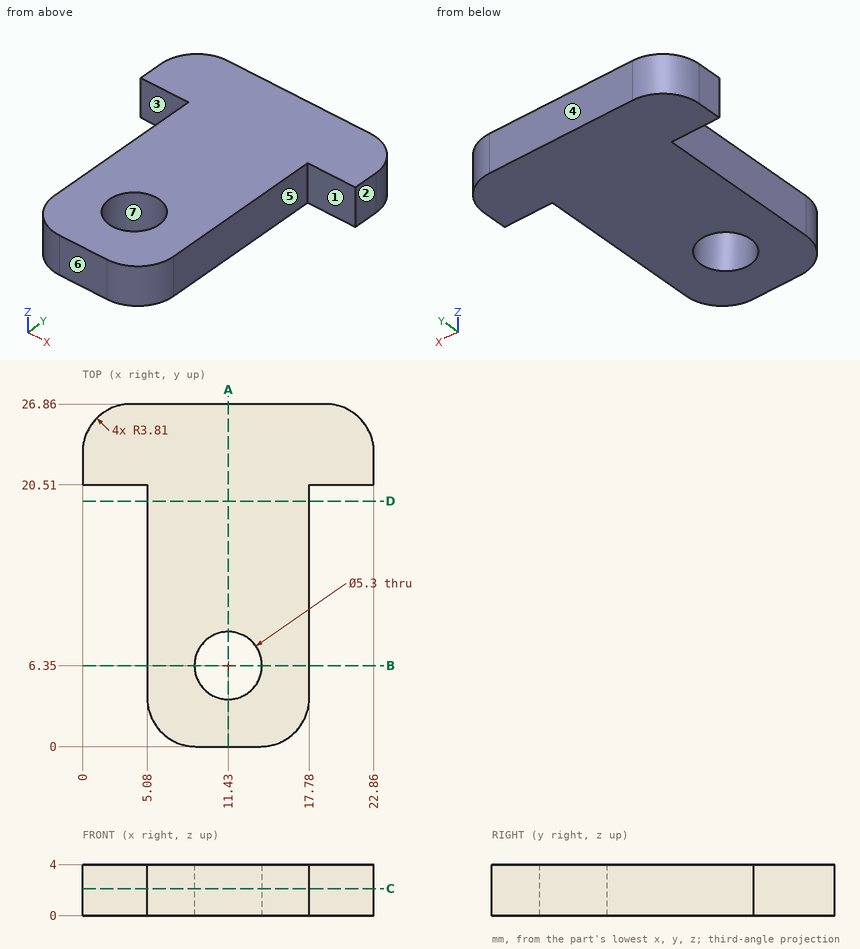
Can you work these out from the drawing? Everything is in mm from the part's minimum corner. A direction names the side the tool comes from. Give positions to 0.01 mm unless a question says otherwise; leave off trailing zeros. Order: outer loops, then holes, each group sorted by start corner. A loop starts at its lowest first (then second) coordinate and runs counter-clockwise, first axis right, second up. Notation, with made-up numbers: M 6,18.5 L 22,18.5 A10 cw 22,27.5 Z; hole C -38.75,72.5 d6. An arc over 180 degrees is marked long. Write item = value, one per line. Start each with the question number.
Q1. Suppose I cut it at B-B (y = 6.35). Write out the boundary of the cut face in (x, z).
Q2. For the marked faces 1, 2 and 3, which set-ups out of +Z, -Z, +X, -X, +Y, -Y let a thin tool reach every point of the face, with its end or its side?
Q3. We'd pull the mould along Y, two halves only. Please class the marked faces 4, 5, 6 and 7: pulls with the +Y half, pulls with the -Y half, needs draft (parallel to the pull), parting line crosses it, or undercut.
Q4. Will these pins go through, and if not, where does the flat tip stop? pin 1 Ø2 at (y, z) = (15.5, 2.5) entering from -X; pin 2 Ø2 at (x, z) = (2.5, 1.5) entering from -Y.
Q5. Suppose I cut it at C-C (z = 2.1). Write out the boundary of the cut face in (x, y), plus the area to 3 significant figures.
Q6. I need wall thicknesses on probe 1 along Y at (x, z) = (11.43, 1.05); probe 2 along X at (y, z) = (20, 2); probe 3 along Y at (x, z) = (4.75, 1.95). Which ranges of each line are inside material? Lowest first, please. Write a range as [from, to].
Q7. Suppose I cut it at A-A (x = 11.43). Write out the boundary of the cut face in (y, z), plus the area to 3 significant figures.
Q8. Suppose I cut it at D-D (y = 19.25). Write out the boundary of the cut face in (x, z).
Check result:
q1.outline = M 5.08,0 L 8.78,0 L 8.78,4 L 5.08,4 Z; M 14.08,0 L 17.78,0 L 17.78,4 L 14.08,4 Z
q2.face_1 = +Z, -Z, +X, -Y
q2.face_2 = +Z, -Z, +X, +Y, -Y
q2.face_3 = +Z, -Z, -X, -Y
q3.face_4 = pulls with the +Y half
q3.face_5 = needs draft
q3.face_6 = pulls with the -Y half
q3.face_7 = undercut
q4.pin_1 = 5.08
q4.pin_2 = 20.51
q5.outline = M 0,20.51 L 5.08,20.51 L 5.08,3.81 A3.81 ccw 8.89,0 L 13.97,0 A3.81 ccw 17.78,3.81 L 17.78,20.51 L 22.86,20.51 L 22.86,23.05 A3.81 ccw 19.05,26.86 L 3.81,26.86 A3.81 ccw 0,23.05 Z; hole C 11.43,6.35 d5.3
q5.area = 371 mm2
q6.probe_1 = [0, 3.7], [9, 26.86]
q6.probe_2 = [5.08, 17.78]
q6.probe_3 = [20.51, 26.86]
q7.outline = M 0,0 L 3.7,0 L 3.7,4 L 0,4 Z; M 9,0 L 26.86,0 L 26.86,4 L 9,4 Z
q7.area = 86.2 mm2
q8.outline = M 5.08,0 L 17.78,0 L 17.78,4 L 5.08,4 Z
